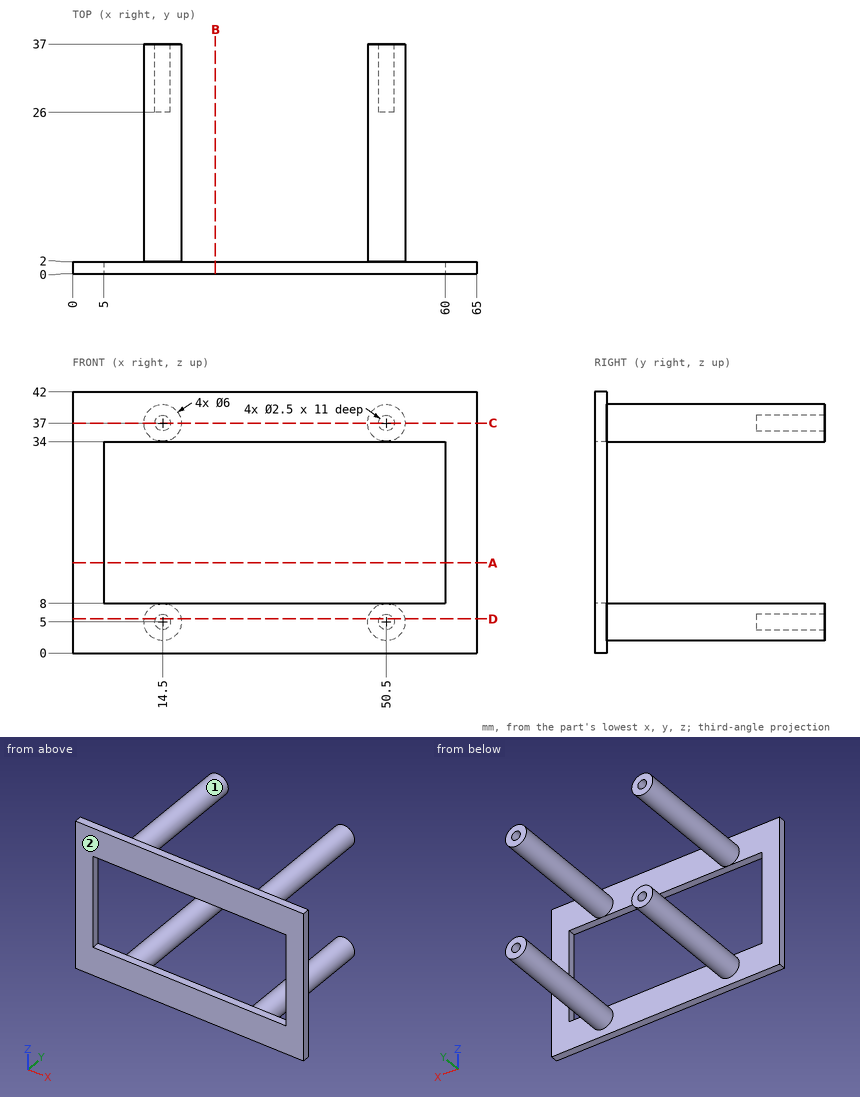
Design review of the part shown in the three views and the two pictorial views. Dimensions are in mm from the part's minimum x, y and z. Give positions to 0.01 mm unless a question says otherwise; leave off trailing zeros. Order: outer loops, then holes, each group sorted by start corner. A loop starts at its lowest first (then second) coordinate and runs counter-clockwise, first axis right, second up. Notation, with made-up numbers: M 73,70 L 126,70 A7 cw 126,81 Z; hole C -1.5,80 d3. An arc over 180 degrees is marked long. Answer in a Markdown table with one row per item. Add a question column.
(1) Consider section C-C on z = 37. State the section outline as (x, y) points.
(2) Mouldability with a two-part tool opening along Z and no side actions: class the marked faces 1 and 2 as +Z half, -Z half, draft (parallel to the pull), parting line (faces both ways), or undercut.
(3) Consider section A-A on z = 14.5. State the section outline as (x, y) points.
(4) For pin 1 (6 mm diameter, centred on y = 6.5, z = 29, fed in from +X); pin 2 (3 mm diameter, centred on x = 47.5, y = 27.5, fed in from +Z); pin 3 (2 mm diameter, centred on x = 50.5, z = 5, fed in from +Y), all flat-tipped, find the tip position at first contact; note any pin that passes through.
(5) Consider section D-D on z = 5.5. State the section outline as (x, y) points, and give its area (3 significant figures).
(6) Consider section B-B on x = 23. State the section outline as (y, z) points, and give its area (3 significant figures).
(7) Wall thickness on probe 1 along X at (y, z) = (28, 37); probe 2 along Z at (x, y) = (14, 33); probe 3 along Y at (x, z) = (4, 27): over which ranges is each line inside the solid? List them lowest first. Write a range as [from, to].
Evaluation:
| question | item | result |
|---|---|---|
| 1 | outline | M 0,0 L 65,0 L 65,2 L 53.5,2 L 53.5,37 L 51.75,37 L 51.75,26 L 49.25,26 L 49.25,37 L 47.5,37 L 47.5,2 L 17.5,2 L 17.5,37 L 15.75,37 L 15.75,26 L 13.25,26 L 13.25,37 L 11.5,37 L 11.5,2 L 0,2 Z |
| 2 | face 1 | undercut |
| 2 | face 2 | draft |
| 3 | outline | M 0,0 L 5,0 L 5,2 L 0,2 Z; M 60,0 L 65,0 L 65,2 L 60,2 Z |
| 4 | pin 1 | passes through |
| 4 | pin 2 | stops at z = 39.6 |
| 4 | pin 3 | stops at y = 26 |
| 5 | outline | M 0,0 L 65,0 L 65,2 L 53.46,2 L 53.46,37 L 51.65,37 L 51.65,26 L 49.35,26 L 49.35,37 L 47.54,37 L 47.54,2 L 17.46,2 L 17.46,37 L 15.65,37 L 15.65,26 L 13.35,26 L 13.35,37 L 11.54,37 L 11.54,2 L 0,2 Z |
| 5 | area | 494 mm^2 |
| 6 | outline | M 0,0 L 2,0 L 2,8 L 0,8 Z; M 0,34 L 2,34 L 2,42 L 0,42 Z |
| 6 | area | 32.0 mm^2 |
| 7 | probe 1 | x = [11.5, 13.25], [15.75, 17.5], [47.5, 49.25], [51.75, 53.5] |
| 7 | probe 2 | z = [2.04, 3.85], [6.15, 7.96], [34.04, 35.85], [38.15, 39.96] |
| 7 | probe 3 | y = [0, 2] |
